Answer from the drawing. Dimensions are ordinates in mm from the lowest x, y and z of the part. A direction names the side the tool comes from. Coordinates: 2 decimals unless noted, no trailing zeros. Order: outer loops, then holes, each group sorted by start corner. A loop starts at its lowest first (then second) coordinate and runs counter-clockwise, first axis right, second up. Notation, with made-up numbers: (58.25, 4.5) - (68.25, 4.5) arc R20 cw to (68.25, 14.5) - close; hole circle Ø10 at (12.25, -3.5). An arc over 180 degrees is marked (long way). One line per item, written item: value. Start each with the question number.
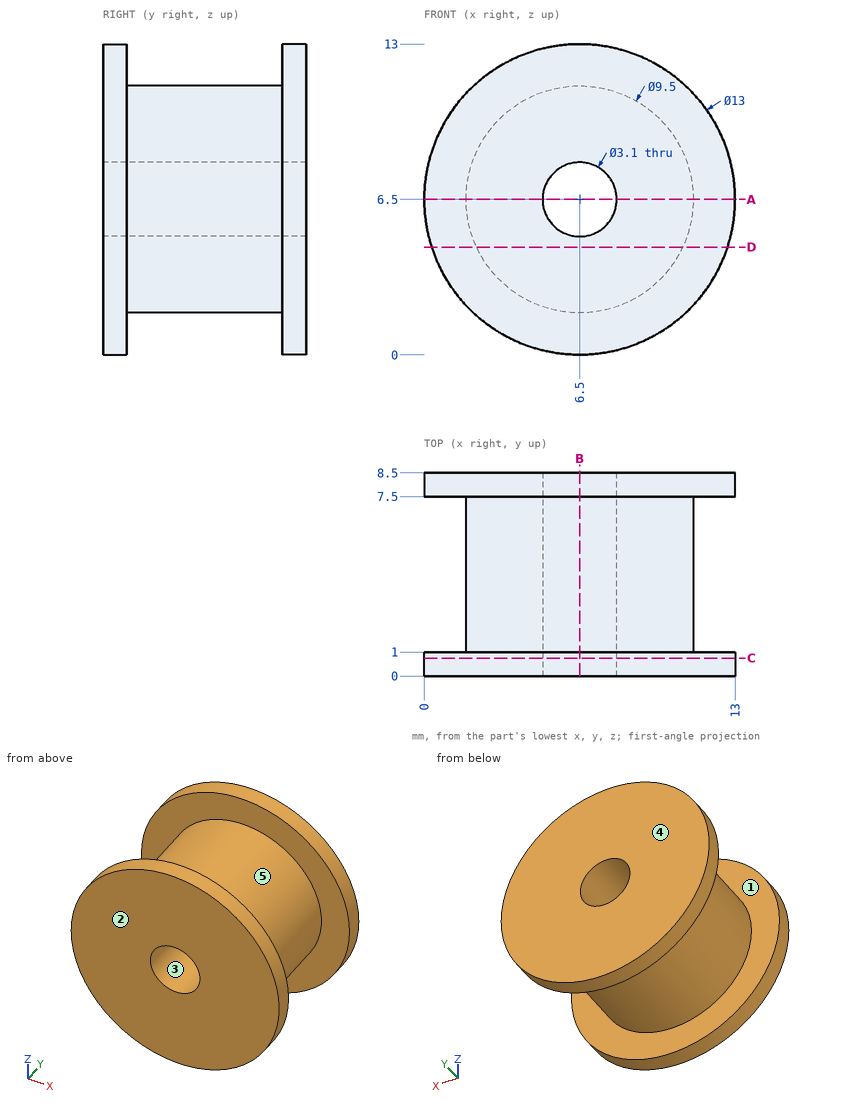
(1) A flat-ended cylindrical pin translates along its axis: pin 1 Ø2 at (x, y) = (11, 1.5) entering from -Z. Find the tip coordinate at first contact, or state that the pin passes through.
(2) The part is cut by section C-C on y = 0.75. Determine the outline of the cut face in (x, z), plus the area to 3 significant figures.
(3) The part is cut by section D-D on z = 4.5. Determine the outline of the cut face in (x, y).
(4) The part is cut by section B-B on x = 6.5. Determine the outline of the cut face in (y, z).
(5) Consider probe 1 along Z at (x, y) = (6.5, 4); probe 2 along Y at (x, z) = (9, 2.25); probe 3 along X at (y, z) = (3.25, 5.5). Determine where each line is inside the solid, lowest interval first.
(6) For a pull along Y with two mould halves and no side action, classify the marked faces 3, 4 and 5 as pulls with the +Y half, pulls with the -Y half, needs draft (parallel to the pull), parting line crosses it, or undercut.
(7) The part is cut by section A-A on z = 6.5. Determine the outline of the cut face in (x, y).
(8) For the marked faces 1 and 2, determine the directions among +Z, -Z, +X, -X, +Y, -Y from which every point of the face is accessible in a straight line to the end or side of a thin tool.
Completed:
1. pin 1: stops at z = 1.11
2. outline: circle Ø13 at (6.5, 6.5); hole circle Ø3.1 at (6.5, 6.5)
2. area: 125 mm2
3. outline: (0.32, 0) - (12.68, 0) - (12.68, 1) - (10.81, 1) - (10.81, 7.5) - (12.68, 7.5) - (12.68, 8.5) - (0.32, 8.5) - (0.32, 7.5) - (2.19, 7.5) - (2.19, 1) - (0.32, 1) - close
4. outline: (0, 0) - (1, 0) - (1, 1.75) - (7.5, 1.75) - (7.5, 0) - (8.5, 0) - (8.5, 4.95) - (0, 4.95) - close; (0, 8.05) - (8.5, 8.05) - (8.5, 13) - (7.5, 13) - (7.5, 11.25) - (1, 11.25) - (1, 13) - (0, 13) - close
5. probe 1: z = 1.75 to 4.95, 8.05 to 11.25
5. probe 2: y = 0 to 1, 7.5 to 8.5
5. probe 3: x = 1.86 to 5.32, 7.68 to 11.14
6. face 3: needs draft
6. face 4: pulls with the +Y half
6. face 5: undercut
7. outline: (0, 0) - (4.95, 0) - (4.95, 8.5) - (0, 8.5) - (0, 7.5) - (1.75, 7.5) - (1.75, 1) - (0, 1) - close; (8.05, 0) - (13, 0) - (13, 1) - (11.25, 1) - (11.25, 7.5) - (13, 7.5) - (13, 8.5) - (8.05, 8.5) - close
8. face 1: none
8. face 2: +Z, -Z, +X, -X, -Y
